Check sheet for the modelled part. Datum: model origin and axes. Units: mm. Round coordinates to 2 decimals unless told otherwise and drop trailing zeros. Loops run counter-clockwise (first coordinate to the right, second up) from the corner with the lowest first, then second, coordinate; pieces in that order, holes last. Notation, with made-up numbers: (63.25, 33.5) - (99.25, 33.5) arc R12 ccw to (99.25, 56.5) - close; hole circle Ø1 at (16.25, -29.5). An arc over 180 degrees is marked (long way). Put each result on its own line as item: value.
```python
from build123d import *

# Parameters (mm, degrees)
SKETCH2_R           = 5
SKETCH2_R_2         = 6
BOSS_EXTRUDE1_DEPTH = 10


with BuildPart() as part:
    # Sketch2 → Boss-Extrude1 (new body)
    with BuildSketch(Plane.XY):
        with BuildLine():
            Line((-737.317762878, -23.619861577), (127.964701196, -23.619861577))
            ThreePointArc((127.964701196, -23.619861577), (135.035769008, -20.690929389), (137.964701196, -13.619861577))
            Line((137.964701196, -13.619861577), (137.964701196, 261.380138423))
            ThreePointArc((137.964701196, 261.380138423), (135.035769008, 268.451206235), (127.964701196, 271.380138423))
            Line((127.964701196, 271.380138423), (-688.827843183, 271.380138423))
            ThreePointArc((-688.827843183, 271.380138423), (-695.25571928, 269.040582854), (-698.675920713, 263.116620199))
            Line((-698.675920713, 263.116620199), (-747.165840408, -11.883379801))
            ThreePointArc((-747.165840408, -11.883379801), (-744.978207309, -20.047737674), (-737.317762878, -23.619861577))
        make_face()
        with Locations(Location((122.964701196, 256.380138423, 0), (0, 0, 180))):
            Circle(SKETCH2_R, mode=Mode.SUBTRACT)
        with Locations((-520.685298804, 35.380138423)):
            Circle(SKETCH2_R_2, mode=Mode.SUBTRACT)
        with Locations(Location((122.964701196, 26.380138423, 0), (0, 0, 180))):
            Circle(SKETCH2_R, mode=Mode.SUBTRACT)
        with Locations((-551.435298804, 256.380138423)):
            Circle(SKETCH2_R, mode=Mode.SUBTRACT)
        with Locations(Location((-456.185298804, 35.380138423, 0), (0, 0, 180))):
            Circle(SKETCH2_R_2, mode=Mode.SUBTRACT)
        with Locations((-424.685298804, 35.380138423)):
            Circle(SKETCH2_R_2, mode=Mode.SUBTRACT)
        with Locations(Location((-360.185298804, 35.380138423, 0), (0, 0, 180))):
            Circle(SKETCH2_R_2, mode=Mode.SUBTRACT)
        with Locations((-328.685298804, 35.380138423)):
            Circle(SKETCH2_R_2, mode=Mode.SUBTRACT)
        with Locations(Location((-264.185298804, 35.380138423, 0), (0, 0, 180))):
            Circle(SKETCH2_R_2, mode=Mode.SUBTRACT)
        with Locations((-232.685298804, 35.380138423)):
            Circle(SKETCH2_R_2, mode=Mode.SUBTRACT)
        with Locations(Location((-168.185298804, 35.380138423, 0), (0, 0, 180))):
            Circle(SKETCH2_R_2, mode=Mode.SUBTRACT)
        with Locations((-136.685298804, 35.380138423)):
            Circle(SKETCH2_R_2, mode=Mode.SUBTRACT)
        with Locations(Location((-72.185298804, 35.380138423, 0), (0, 0, 180))):
            Circle(SKETCH2_R_2, mode=Mode.SUBTRACT)
        with Locations((-551.435298804, 26.380138423)):
            Circle(SKETCH2_R, mode=Mode.SUBTRACT)
        with Locations((-40.685298804, 35.380138423)):
            Circle(SKETCH2_R_2, mode=Mode.SUBTRACT)
        with Locations(Location((23.814701196, 35.380138423, 0), (0, 0, 180))):
            Circle(SKETCH2_R_2, mode=Mode.SUBTRACT)
        with BuildLine():
            Line((-531.435298804, 46.380138423), (37.064561069, 46.380138423))
            ThreePointArc((37.064561069, 46.380138423), (44.135628881, 49.309070611), (47.064561069, 56.380138423))
            Line((47.064561069, 56.380138423), (47.064561069, 136.380138423))
            ThreePointArc((47.064561069, 136.380138423), (44.135628881, 143.451206235), (37.064561069, 146.380138423))
            Line((37.064561069, 146.380138423), (-531.435298804, 146.380138423))
            ThreePointArc((-531.435298804, 146.380138423), (-538.506366616, 143.451206235), (-541.435298804, 136.380138423))
            Line((-541.435298804, 136.380138423), (-541.435298804, 56.380138423))
            ThreePointArc((-541.435298804, 56.380138423), (-538.506366616, 49.309070611), (-531.435298804, 46.380138423))
        make_face(mode=Mode.SUBTRACT)
    extrude(amount=BOSS_EXTRUDE1_DEPTH)


solid = part.part
```
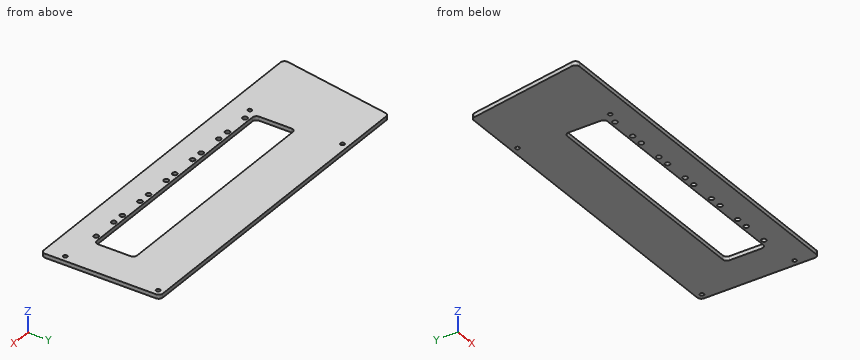
Item 1: Section check A-A on x = -13.5. Enter the section's corners in (y, z), then the cut area to 3 significant figures.
Filled sheet:
outline: (-23.62, 0) - (46.38, 0) - (46.38, 10) - (-23.62, 10) - close; (146.38, 0) - (271.38, 0) - (271.38, 10) - (146.38, 10) - close
area: 1,950 mm²
Item 2: Section check C-C on y = 219.5. Enter the section's corners in (x, z).
Filled sheet:
outline: (-706.37, 0) - (137.96, 0) - (137.96, 10) - (-706.37, 10) - close
Item 3: Thickness scan on line 1 (Y direction, x = -487.5, z = 3.5); line 2 (Y direction, x = -163, z = 4.25); line 3 (X direction, y = 256.5, z = 1.5). Record the ranges inside material, lowest first. Write a range as from..to.
Filled sheet:
line 1: -23.62..46.38, 146.38..271.38
line 2: -23.62..32.36, 38.4..46.38, 146.38..271.38
line 3: -699.84..-556.43, -546.44..117.97, 127.96..137.96
Item 4: Go/stop test with flat-tipped pins: pin 1 (15.5 mm diameter, centred on x = -136.69, y = 35.38, fed in from +Z); pin 2 (1.5 mm diameter, centred on y = 167, z = 8.5, fed in from -X); pin 3 (9.5 mm diameter, centred on x = -328.69, y = 35.38, fed in from -Z). Record where each tip stops, or that it passes through.
Filled sheet:
pin 1: z = 10
pin 2: x = -715.76
pin 3: through
Item 5: Section check B-B on z = 7.5. Count the separate pieces of the cut face and the enclosed holes in it, then the cut area to 3 significant figures.
Filled sheet:
separate pieces: 1
enclosed holes: 17
area: 194,000 mm²
